Source: CAD feature listing. Evaluate the final solid. Frame: model axes, mm. Face numbers are marked on the shaded views. A direction names the side the tool comes from. Round coordinates to 2 decimals unless told otherwise and drop trailing zeros. Loops run counter-clockwise (first coordinate to the right, second up) from the corner with the lowest first, then second, coordinate; pieces in that order, holes last. Notation, with made-up numbers: (-29, 21.25) -> (-25, 21.25) arc R15 ccw to (-25, 50.25) -> close; hole circle Ø6 at (-10, 34.25). An arc over 180 degrees is marked (long way). Put each result on its own line as item: value. Start each with the question number.
1. Cut plane A-A (x = -25.5). Return the cut outline in (y, z), then the cut area to 3 significant figures.
2. Contact query for flat-ended pins moving along their axis: pin 1 (8 mm diameter, centred on x = 8.5, y = 16, fed in from +Z); pin 2 (8 mm diameter, centred on y = 0.5, z = 32, fed in from +X); pin 3 (10.5 mm diameter, centred on y = 18.5, z = 17.5, fed in from +X). Output: stop coordinate, or through.
3. Cut plane D-D (z = 39). Return the cut outline in (x, y).
4. Cut plane B-B (y = 25). Return the cut outline in (x, z).
5. Set-up query: the marked faces 4, 5 and 6. Return all of +Z, -Z, +X, -X, +Y, -Y with unobstructed straight access to the full face (end or side cutting, diameter ignored); none if empty.
6. Draft query along Z for the marked faces 1, 2 and 3. Return one class per face: pulls with the +Z half, pulls with the -Z half, needs draft (parallel to the pull), parting line crosses it, or undercut.
7. Material intervals for L1, parallel to Y at x = -25.5, z = -14.8; L2, parallel to Z at x = -13, y = 0; L3, parallel to Y at x = 9, z = 29.5, sorted ascending.
8. Cut plane C-C (x = 64.5). Return the cut outline in (y, z).
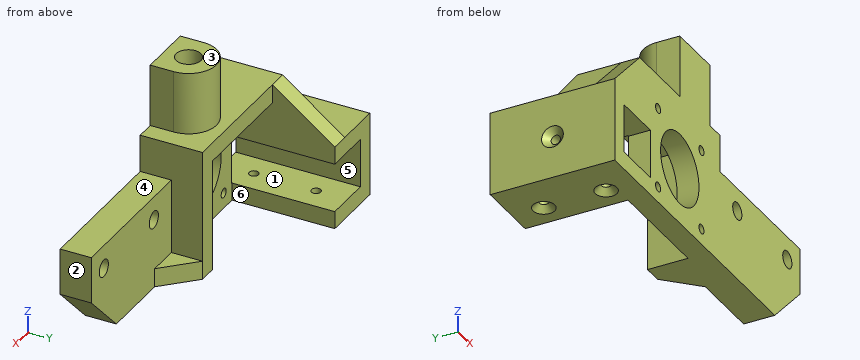
```python
from build123d import *

# Parameters (mm, degrees)
F0_R        = 1.5
F0_W        = 15
F0_H        = 15
F0_R_2      = 11.5
F1_DEPTH    = 5
F3_DEPTH    = 35
F5_DEPTH    = 20
F6_R        = 1.5
F7_DEPTH    = 6.001
F9_DEPTH    = 6
F11_DEPTH   = 6
F12_R       = 1.5
F13_DEPTH   = 6.001
F14_W       = 20
F14_H       = 42
F15_DEPTH   = 6
F16_R       = 2.75
F17_DEPTH   = 10
F19_DEPTH   = 6
F20_SIZE    = 2
F21_W       = 15.7
F21_H       = 15.7
F22_DEPTH   = 40.001
F1_FACE_R   = 1.5
F1_FACE_R_2 = 11.5
F23_DEPTH   = 2
F24_R       = 4
F25_DEPTH   = 20


with BuildPart() as f1:
    # F0 (on Front) → F1 (new body)
    with BuildSketch(Plane.XZ):
        Polygon((18, -18), (18, 18), (-18, 18), (-18, 9), (-33, 9), (-39, 9), (-39, -18), (-33, -18), (-18, -18), align=None)
        with Locations((-13, -13)):
            Circle(F0_R, mode=Mode.SUBTRACT)
        with Locations((-25.5, -4.5)):
            Rectangle(F0_W, F0_H, mode=Mode.SUBTRACT)
        with Locations((13, -13)):
            Circle(F0_R, mode=Mode.SUBTRACT)
        with Locations((-13, 13)):
            Circle(F0_R, mode=Mode.SUBTRACT)
        Circle(F0_R_2, mode=Mode.SUBTRACT)
        with Locations((13, 13)):
            Circle(F0_R, mode=Mode.SUBTRACT)
    extrude(amount=F1_DEPTH)

    # F2 (on face) → F3 (join)
    with BuildSketch(Plane(origin=(0, 0, 0), x_dir=(-1, 0, 0), z_dir=(0, 1, 0))):
        Polygon((18, 9), (18, 3), (33, 3), (33, -12), (18, -12), (18, -18), (39, -18), (39, 9), align=None)
    extrude(amount=F3_DEPTH)

    # F4 (on face) → F5 (join)
    with BuildSketch(Plane.XZ.offset(5)):
        Polygon((-24, 9), (-18, 9), (-18, 18), (18, 18), (18, 24), (-24, 24), align=None)
    extrude(amount=-F5_DEPTH)

    # F6 (on face) → F7 (cut, through all)
    with BuildSketch(Plane.YZ.offset(-33)):
        with Locations((15, -4.5)):
            Circle(F6_R)
    extrude(amount=-F7_DEPTH, mode=Mode.SUBTRACT)

    # F8 (on face) → F9 (join, through all)
    with BuildSketch(Plane(origin=(-24, 0, 0), x_dir=(0, -1, 0), z_dir=(-1, 0, 0))):
        Polygon((-15, 9), (-15, 24), (-35, 9), align=None)
    extrude(amount=-F9_DEPTH)

    # F10 (on face) → F11 (join)
    with BuildSketch(Plane.XZ.offset(5)):
        Polygon((-24, 9), (-24, 24), (-39, 9), align=None)
    extrude(amount=-F11_DEPTH)

    # F12 (on face) → F13 (cut, through all)
    with BuildSketch(Plane.XY.offset(-12)):
        with Locations((-25.5, 5)):
            Circle(F12_R)
        with Locations((-25.5, 25)):
            Circle(F12_R)
    extrude(amount=-F13_DEPTH, mode=Mode.SUBTRACT)

    # F14 (on face) → F15 (join)
    with BuildSketch(Plane.YZ.offset(18)):
        with Locations((5, 3)):
            Rectangle(F14_W, F14_H)
    extrude(amount=F15_DEPTH)

    # F16 (on face) → F17 (join)
    with BuildSketch(Plane.XZ.offset(5)):
        Polygon((24, 12), (24, -18), (57, -18), (72, -3), (72, 12), align=None)
        with Locations((34.5, 4.5)):
            Circle(F16_R, mode=Mode.SUBTRACT)
        with Locations((64.5, 4.5)):
            Circle(F16_R, mode=Mode.SUBTRACT)
    extrude(amount=-F17_DEPTH)

    # F18 (on face) → F19 (join, through all)
    with BuildSketch(Plane(origin=(0, 0, -18), x_dir=(1, 0, 0), z_dir=(0, 0, -1))):
        Polygon((34, -5), (24, -5), (24, -15), align=None)
    extrude(amount=-F19_DEPTH)

    # F20
    f20_edges = [f1.edges().sort_by_distance(p)[0] for p in [
        (-39, 13.5, -4.5),
        (-27, 5, -18),
        (-27, 25, -18),
    ]]
    chamfer(f20_edges, length=F20_SIZE)

    # F21 (on face) → F22 (cut, through all)
    with BuildSketch(Plane.XZ.offset(5)):
        with Locations((-25.5, -4.5)):
            Rectangle(F21_W, F21_H)
    extrude(amount=-F22_DEPTH, mode=Mode.SUBTRACT)

    # F1_face (on face) → F23 (join)
    with BuildSketch(Plane(origin=(-8.726816, 0, -1.288675), x_dir=(1, 0, 0), z_dir=(0, 1, 0))):
        Polygon((-9.273184, 16.711325), (-9.273184, 11.061325), (-8.923184, 11.061325), (-8.923184, -4.638675), (-9.273184, -4.638675), (-9.273184, -19.288675), (26.726816, -19.288675), (26.726816, 16.711325), align=None)
        with Locations((-4.273184, 11.711325)):
            Circle(F1_FACE_R, mode=Mode.SUBTRACT)
        with Locations((21.726816, 11.711325)):
            Circle(F1_FACE_R, mode=Mode.SUBTRACT)
        with Locations((-4.273184, -14.288675)):
            Circle(F1_FACE_R, mode=Mode.SUBTRACT)
        with Locations((8.726816, -1.288675)):
            Circle(F1_FACE_R_2, mode=Mode.SUBTRACT)
        with Locations((21.726816, -14.288675)):
            Circle(F1_FACE_R, mode=Mode.SUBTRACT)
    extrude(amount=F23_DEPTH)

    # F24 (on face) → F25 (join)
    with BuildSketch(Plane.XY.offset(24)):
        with BuildLine():
            Line((0, 2.5), (0, -5))
            Line((0, -5), (18, -5))
            Line((18, -5), (18, 2.5))
            ThreePointArc((18, 2.5), (9, 11.5), (0, 2.5))
        make_face()
        with Locations((9, 2.5)):
            Circle(F24_R, mode=Mode.SUBTRACT)
    extrude(amount=F25_DEPTH)


solid = f1.part
```
Solution:
1. outline: (-5, -18) -> (1.5, -18) -> (3.5, -16) -> (3.5, -12.35) -> (-5, -12.35) -> close; (-5, 3.35) -> (35, 3.35) -> (35, 9) -> (1, 9) -> (1, 22.5) -> (-5, 22.5) -> close; (6.5, -16) -> (8.5, -18) -> (21.5, -18) -> (23.5, -16) -> (23.5, -12.35) -> (6.5, -12.35) -> close; (26.5, -16) -> (28.5, -18) -> (35, -18) -> (35, -12.35) -> (26.5, -12.35) -> close
1. area: 491 mm^2
2. pin 1: stops at z = 24
2. pin 2: stops at x = 18
2. pin 3: stops at x = 24
3. outline: (0, -5) -> (18, -5) -> (18, 2.5) arc R9 ccw to (0, 2.5) -> close; hole circle Ø8 at (9, 2.5)
4. outline: (-39, -18) -> (-29, -18) -> (-27, -16) -> (-27, -12.35) -> (-33.35, -12.35) -> (-33.35, 3.35) -> (-18, 3.35) -> (-18, 16.5) -> (-24, 16.5) -> (-24, 9) -> (-39, 9) -> close; (-24, -16) -> (-22, -18) -> (-18, -18) -> (-18, -12.35) -> (-24, -12.35) -> close
5. face 4: +Z, +X, +Y, -Y
5. face 5: +Y, -Y
5. face 6: -Z, +Y
6. face 1: undercut
6. face 2: needs draft
6. face 3: pulls with the +Z half
7. L1: y = -5 to 3.5, 6.5 to 23.5, 26.5 to 35
7. L2: z = -18 to -14.5, -11.5 to 11.5, 14.5 to 24
7. L3: y = -5 to -1.5, 6.5 to 11.5
8. outline: (-5, -10.5) -> (5, -10.5) -> (5, 1.75) -> (-5, 1.75) -> close; (-5, 7.25) -> (5, 7.25) -> (5, 12) -> (-5, 12) -> close
